Can you work these out from the model? Positions are in its coordinate system, mm. Round coordinates to 2 decimals unless told otherwise and drop trailing zeros. Loops run counter-clockwise (first coordinate to the right, second up) from the corner with the lowest first, then second, coordinate; pieces in that order, holes last.
from build123d import *

# Parameters (mm, degrees)
BASE_FLANGE1_DEPTH              = 2
M6X1_0_TAPPED_HOLE1_D           = 5
M6X1_0_TAPPED_HOLE1_DEPTH       = 15
M6X1_0_TAPPED_HOLE1_CSINK_D     = 6.05
M6X1_0_TAPPED_HOLE1_CSINK_ANGLE = 90
M6X1_0_TAPPED_HOLE1_TIP         = 1.502151548
FILLET1_R                       = 2


# Sheet-metal steps are written as plain solids
with BuildPart() as part:
    # Sketch1 → Base-Flange1 (new body)
    with BuildSketch(Plane.XY):
        Polygon((13.346640495, -13.346640495), (45.577783105, 18.884502115), (144.559502115, 18.884502115), (144.559502115, 56.634502115), (83.327783105, 56.634502115), (88.865644726, 62.172363736), (62.172363736, 88.865644726), (-13.346640495, 13.346640495), align=None)
    extrude(amount=-BASE_FLANGE1_DEPTH)

    # M6x1.0 Tapped Hole1
    with Locations(Plane.XY):
        with Locations((56.639253173, 56.639253173), (18.879751058, 18.879751058), (113.94364261, 37.759502115)):
            CounterSinkHole(M6X1_0_TAPPED_HOLE1_D / 2, M6X1_0_TAPPED_HOLE1_CSINK_D / 2, depth=M6X1_0_TAPPED_HOLE1_DEPTH, counter_sink_angle=M6X1_0_TAPPED_HOLE1_CSINK_ANGLE)
            with Locations((0, 0, -(M6X1_0_TAPPED_HOLE1_DEPTH + M6X1_0_TAPPED_HOLE1_TIP / 2))):  # 118° drill point
                Cone(0, M6X1_0_TAPPED_HOLE1_D / 2, M6X1_0_TAPPED_HOLE1_TIP, mode=Mode.SUBTRACT)

    # Fillet1
    fillet1_edges = [part.edges().sort_by_distance(p)[0] for p in [
        (-13.346640495, 13.346640495, -1),
        (62.172363736, 88.865644726, -1),
        (88.865644726, 62.172363736, -1),
        (83.327783105, 56.634502115, -1),
        (144.559502115, 56.634502115, -1),
        (144.559502115, 18.884502115, -1),
        (45.577783105, 18.884502115, -1),
        (13.346640495, -13.346640495, -1),
    ]]
    fillet(fillet1_edges, radius=FILLET1_R)


solid = part.part
(1) If I drill on line 1 (Y direction, x = 126, z = -1.65); line 2 (Y direction, x = 19, z = -1.05); line 3 (X direction, y = 54.5, z = -1.3), over which ranges is the centre line in solid material (lowest first)?
Worked answers:
line 1: y = 18.88 to 56.63
line 2: y = -7.69 to 16.38, 21.38 to 45.69
line 3: x = 27.81 to 55.35, 57.93 to 144.56
(2) If we section it at A-A, the plane z = -0.95: List the corners of the cut face in (x, y) for me, then the cut area to 3 significant figures.
Worked answers:
outline: (-11.93, 11.93) - (11.93, -11.93) arc R2 ccw to (14.76, -11.93) - (44.99, 18.3) arc R2 cw to (46.41, 18.88) - (142.56, 18.88) arc R2 ccw to (144.56, 20.88) - (144.56, 54.63) arc R2 ccw to (142.56, 56.63) - (88.16, 56.63) arc R2 cw to (86.74, 60.05) - (87.45, 60.76) arc R2 ccw to (87.45, 63.59) - (63.59, 87.45) arc R2 ccw to (60.76, 87.45) - (-11.93, 14.76) arc R2 ccw to start; hole circle Ø5 at (18.88, 18.88); hole circle Ø5 at (56.64, 56.64); hole circle Ø5 at (113.94, 37.76)
area: 7,000 mm2
(3) Will this pin go through, and if not, where does the flat tip stop? P1, Ø3, axis at x = 113.94, y = 37.76, coming from the -Z side.
Worked answers:
P1: passes through
(4) If we mould it in two halves opening along Y, with no side actions, what happens to faces 1 (the cylindrical face through (20.72, 20.57, -1.27)), 2 (the flat face through (65, 38, -2)), 3 (the flat face through (29.665, 2.972, -0.986))? For each: released by +Y, released by -Y, zero draft, split by the parting line, or undercut.
Worked answers:
face 1: undercut
face 2: zero draft
face 3: released by -Y
(5) If we section it at B-B, the plane x = 135.5: List the corners of the cut face in (y, z) for me.
Worked answers:
outline: (18.88, -2) - (56.63, -2) - (56.63, 0) - (18.88, 0) - close
(6) If we section it at C-C, the plane y = 2: List the corners of the cut face in (x, z) for me, then the cut area to 3 significant figures.
Worked answers:
outline: (-2, -2) - (28.69, -2) - (28.69, 0) - (-2, 0) - close
area: 61.4 mm2
